Verification items for the finished model (mm, model axes). A direction names the side the tool comes from. Round coordinates to 2 decimals unless told otherwise and drop trailing zeros. Write each loop counter-clockwise with the first axis right and the second up, starting at its lowest first coordinate (ties: lowest second). Pieces come first, ordered by that corner, then holes. Notation, with made-up numbers: (81, -20) - (98, -20) arc R24 ccw to (98, 3) - close; hole circle Ø7 at (16.25, 37.5). An arc over 180 degrees is marked (long way). Answer as a JSON object with one key per item and string values.
Autodesk Inventor part; units mm, degrees
ref_plane "YZ Plane" through (0, 0, 0) normal (1, 0, 0) x (0, 1, 0)
ref_plane "XZ Plane" through (0, 0, 0) normal (0, 1, 0) x (-1, 0, 0)
ref_plane "XY Plane" through (0, 0, 0) normal (0, 0, 1) x (1, 0, 0)
sketch "Sketch1" plane through (0, 0, 0) normal (0, 1, 0) x (-1, 0, 0)
  line L0 (-70, 125) -> (-70, 95)
  line L1 (-70, 95) -> (-45, 95)
  line L2 (-45, 95) -> (0, 50)
  line L3 (0, 50) -> (0, 0)
  line L4 (-70, 125) -> (-45, 125)
  line L5 (-45, 125) -> (30, 50)
  line L6 (30, 50) -> (30, 0)
  line L7 (0, 0) -> (-70, 0) construction
  line L8 (-70, -125) -> (-70, -95)
  line L9 (-70, -95) -> (-45, -95)
  line L10 (-45, -95) -> (0, -50)
  line L11 (0, -50) -> (0, 0)
  line L12 (-70, -125) -> (-45, -125)
  line L13 (-45, -125) -> (30, -50)
  line L14 (30, -50) -> (30, 0)
  line L15 (-42.9289, 100) -> (-65, 100)
  line L16 (-65, 100) -> (-65, 120)
  line L17 (-65, 120) -> (-47.0711, 120)
  line L18 (-47.0711, 120) -> (25, 47.9289)
  line L19 (25, 47.9289) -> (25, 0)
  line L20 (25, 0) -> (25, -47.9289)
  line L21 (25, -47.9289) -> (-47.0711, -120)
  line L22 (-47.0711, -120) -> (-65, -120)
  line L23 (-65, -120) -> (-65, -100)
  line L24 (-65, -100) -> (-42.9289, -100)
  line L25 (-42.9289, -100) -> (5, -52.0711)
  line L26 (5, -52.0711) -> (5, 0)
  line L27 (5, 0) -> (5, 52.0711)
  line L28 (5, 52.0711) -> (-42.9289, 100)
  dimension "d0" = 125
  dimension "d1" = 30
  dimension "d4" = 30
  dimension "d5" = 25
  dimension "d6" = 100
  dimension "d7" = 20
extrude "Extrusion3" add sketch "Sketch1" along normal mid plane 6 contours L4 L5 L6 L14 L13 L12 L8 L9 L10 L11 L3 L2 L1 L0 | L15 L16 L17 L18 L19 L20 L21 L22 L23 L24 L25 L26 L27 L28
extrude "Extrusion4" add sketch "Sketch1" along normal blind 25
sketch "Sketch2" plane through (-30, -3, -50) normal (-1, 0, 0) x (0, 0, 1)
  circle A0 centre (50, 15) radius 6
  point P0 (50, 3)
  dimension "d16" = 12
extrude "Extrusion5" add sketch "Sketch2" along normal blind 2
properties part number "prettylny"
Q1. Section check D-D, the plane y = 0.5. Record the cut outline in (x, z).
Geometry check:
{"outline": "(-30, -50) - (45, -125) - (70, -125) - (70, -95) - (45, -95) - (0, -50) - (0, 50) - (45, 95) - (70, 95) - (70, 125) - (45, 125) - (-30, 50) - close"}
Q2. Material ranges on line 1 along Z through (x, y) = (52.5, -0.75); line 2 along X through (y, z) = (4.5, 7.5); line 3 along Z through (x, y) = (47, 22.75), recorded low to high. Write a range as [from, to].
Geometry check:
{"line 1": "z = [-125, -95], [95, 125]", "line 2": "x = [-30, -25], [-5, 0]", "line 3": "z = [-125, -119.93], [-100, -95], [95, 100], [119.93, 125]"}
Q3. Section check C-C, the plane x = 8. Record the cut outline in (y, z), then the cut area to 3 significant figures.
Geometry check:
{"outline": "(-3, -88) - (25, -88) - (25, -80.93) - (3, -80.93) - (3, -65.07) - (25, -65.07) - (25, -58) - (-3, -58) - close; (-3, 58) - (25, 58) - (25, 65.07) - (3, 65.07) - (3, 80.93) - (25, 80.93) - (25, 88) - (-3, 88) - close", "area": "982 mm2"}
Q4. Release check for a two-part mould opening along X. For faces 1 (the flat face through (-2, 25, 10)), 2 (the flat face through (-25, 14, 1)), 3 (the flat face through (56, 14, 120)), 4 (the flat face through (70, 11, 110)) record: released by +X, released by -X, zero draft, split by the parting line, or undercut.
Geometry check:
{"face 1": "zero draft", "face 2": "undercut", "face 3": "undercut", "face 4": "released by +X"}
Q5. Section check A-A, the plane z = 0. Record the cut outline in (x, y).
Geometry check:
{"outline": "(-32, 6) - (-30, 6) - (-30, -3) - (0, -3) - (0, 25) - (-5, 25) - (-5, 3) - (-25, 3) - (-25, 25) - (-30, 25) - (-30, 18) - (-32, 18) - close"}
Q6. Section check B-B, the plane y = 12. Record the cut outline in (x, z).
Geometry check:
{"outline": "(-32, -6) - (-30, -6) - (-30, -50) - (45, -125) - (70, -125) - (70, -95) - (45, -95) - (0, -50) - (0, 50) - (45, 95) - (70, 95) - (70, 125) - (45, 125) - (-30, 50) - (-30, 6) - (-32, 6) - close; hole (-25, -47.93) - (47.07, -120) - (65, -120) - (65, -100) - (42.93, -100) - (-5, -52.07) - (-5, 52.07) - (42.93, 100) - (65, 100) - (65, 120) - (47.07, 120) - (-25, 47.93) - close"}
Q7. Set-up check for faces 5 (the flat face through (70, 11, -110)), 6 (the flat face through (0, 11, -1)), 7 (the flat face through (-6, 3, 1)), 8 (the flat face through (-32, 12, 0)), 9 (the cylindrical face through (-30.99, 6.05, -0.78)): record each of +Z, -Z, +X, -X, +Y, -Y from which the full face is reachable in a straight line by a thin tool's end or side.
Geometry check:
{"face 5": "+Z, -Z, +X, +Y, -Y", "face 6": "+X, +Y, -Y", "face 7": "+Y", "face 8": "+Z, -Z, -X, +Y, -Y", "face 9": "-X"}
Q8. Gauge pin test, flat ends, axial feed: P1, Ø12, axis at y = 0, z = 7.5, coming from the +X side; P2, Ø4, axis at x = 1.5, y = 20, coming from the +Z side; P3, Ø5, axis at x = 30, y = 17.5, coming from the -Z side. Record the tip position at first contact, or that the pin passes through.
Geometry check:
{"P1": "stops at x = 0", "P2": "stops at z = 83.5", "P3": "stops at z = -112.5"}
